The drawing under review shows one solid part. Ordinate dimensions are in mm from its lowest x, y, z. Give positions to 0.01 mm unless a question says otherwise; leave off trailing zeros. Write each loop counter-clockwise with the first axis right and the second up, starting at its lowest first coordinate (ties: lowest second). Pieces come first, ordered by that corner, then holes. Notation, with made-up numbers: (-1.75, 11.25) -> (34.25, 11.25) arc R20 cw to (34.25, 35.25) -> close; hole circle Ø10 at (44, 4.25). An arc over 180 degrees is marked (long way). Answer as a JSON object with one key per item and string values.
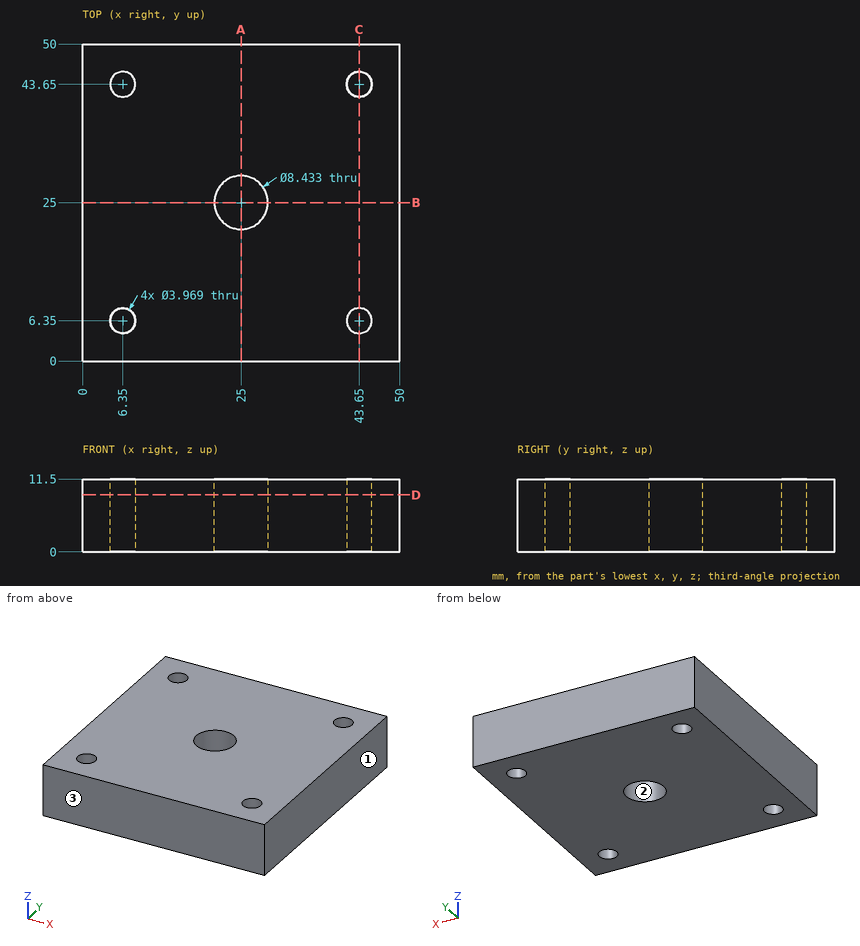
(1) We need section C-C, the plane x = 43.65. State the section outline as (y, z) points.
Here are the results:
{"outline": "(0, 0) -> (4.37, 0) -> (4.37, 11.5) -> (0, 11.5) -> close; (8.33, 0) -> (41.67, 0) -> (41.67, 11.5) -> (8.33, 11.5) -> close; (45.63, 0) -> (50, 0) -> (50, 11.5) -> (45.63, 11.5) -> close"}
(2) For line 1 along X through (y, z) = (6.5, 1); line 2 along X through (y, z) = (7.5, 9), list the stretches that pass through material, from the lowest coordinate up.
Here are the results:
{"line 1": "x = 0 to 4.37, 8.33 to 41.67, 45.63 to 50", "line 2": "x = 0 to 4.73, 7.97 to 42.03, 45.27 to 50"}
(3) Clearance check with flat-ended pins moving along their axes: pin 1 (8 mm diameter, centred on x = 28, y = 41, fed in from -Z); pin 2 (1 mm diameter, centred on x = 44, y = 6.5, fed in from +Z). State where each tip first meets the part, or that it passes through.
Here are the results:
{"pin 1": "stops at z = 0", "pin 2": "passes through"}
(4) We need section D-D, the plane z = 9. State the section outline as (x, y) points, then the cut area to 3 significant figures.
Here are the results:
{"outline": "(0, 0) -> (50, 0) -> (50, 50) -> (0, 50) -> close; hole circle Ø3.97 at (6.35, 6.35); hole circle Ø3.97 at (6.35, 43.65); hole circle Ø8.43 at (25, 25); hole circle Ø3.97 at (43.65, 6.35); hole circle Ø3.97 at (43.65, 43.65)", "area": "2,390 mm²"}
(5) The part is to be moulded in two halves that separate along Y. For the marked faces 1, 2 and 3, say which applies: +Y half, -Y half, draft (parallel to the pull), parting line (faces both ways), or undercut.
Here are the results:
{"face 1": "draft", "face 2": "undercut", "face 3": "-Y half"}
(6) We need section A-A, the plane x = 25. State the section outline as (y, z) points.
Here are the results:
{"outline": "(0, 0) -> (20.78, 0) -> (20.78, 11.5) -> (0, 11.5) -> close; (29.22, 0) -> (50, 0) -> (50, 11.5) -> (29.22, 11.5) -> close"}
